```python
from build123d import *

# Parameters (mm, degrees)
CROQUIS1_R              = 9.5
SALIENTE_EXTRUIR1_DEPTH = 6
CROQUIS2_R              = 1.5
CORTAR_EXTRUIR1_DEPTH   = 6
CROQUIS3_R              = 3
CORTAR_EXTRUIR2_DEPTH   = 6
REDONDEO1_R             = 1


with BuildPart() as part:
    # Croquis1 → Saliente-Extruir1 (new body)
    with BuildSketch(Plane(origin=(0, 0, 0), x_dir=(1, 0, 0), z_dir=(0, 1, 0))):
        with BuildLine():
            ThreePointArc((12.5, 0), (0, 12.5), (-12.5, 0))
            Line((-12.5, 0), (-12.5, -16))
            ThreePointArc((-12.5, -16), (-13.085786438, -17.414213562), (-14.5, -18))
            Line((-14.5, -18), (-20.5, -18))
            Line((-20.5, -18), (-20.5, -21))
            Line((-20.5, -21), (-5.5, -21))
            Line((-5.5, -21), (-5.5, -36))
            Line((-5.5, -36), (5.5, -36))
            Line((5.5, -36), (5.5, -21))
            Line((5.5, -21), (20.5, -21))
            Line((20.5, -21), (20.5, -18))
            Line((20.5, -18), (14.5, -18))
            ThreePointArc((14.5, -18), (13.085786438, -17.414213562), (12.5, -16))
            Line((12.5, -16), (12.5, 0))
        make_face()
        with Locations(Location((0, 0, 0), (0, 0, 270))):
            Circle(CROQUIS1_R, mode=Mode.SUBTRACT)
    extrude(amount=SALIENTE_EXTRUIR1_DEPTH)

    # Croquis2 → Cortar-Extruir1 (cut)
    with BuildSketch(Plane.XY.offset(21)):
        with Locations((-16.5, 3)):
            Circle(CROQUIS2_R)
        with Locations((16.5, 3)):
            Circle(CROQUIS2_R)
    extrude(amount=-CORTAR_EXTRUIR1_DEPTH, mode=Mode.SUBTRACT)

    # Croquis3 → Cortar-Extruir2 (cut)
    with BuildSketch(Plane(origin=(0, 0, 18), x_dir=(-1, 0, 0), z_dir=(0, 0, -1))):
        with Locations((-16.5, 3)):
            Circle(CROQUIS3_R)
        with Locations((16.5, 3)):
            Circle(CROQUIS3_R)
    extrude(amount=CORTAR_EXTRUIR2_DEPTH, mode=Mode.SUBTRACT)

    # Redondeo1
    redondeo1_edges = [part.edges().sort_by_distance(p)[0] for p in [
        (5.5, 3, 36),
        (-5.5, 3, 36),
        (0, 6, 36),
        (0, 0, 36),
    ]]
    fillet(redondeo1_edges, radius=REDONDEO1_R)


solid = part.part
```
Model file for the job. Use its own axes, mm. A direction names the side the tool comes from. Coordinates: 2 decimals unless noted, no trailing zeros. Order: outer loops, then holes, each group sorted by start corner. A loop starts at its lowest first (then second) coordinate and runs counter-clockwise, first axis right, second up. Notation, with made-up numbers: (42, 43) -> (92, 43) arc R15 ccw to (92, 65) -> close; hole circle Ø10 at (-15, 84). An arc over 180 degrees is marked (long way). Return JSON: item names as keys, results as strings.
Item 1: Slice it at B-B (x = 0). Write the cut outline in (y, z), then the cut area to 3 significant figures.
Model answer:
{"outline": "(0, -12.5) -> (6, -12.5) -> (6, -9.5) -> (0, -9.5) -> close; (0, 9.5) -> (6, 9.5) -> (6, 35) arc R1 ccw to (5, 36) -> (1, 36) arc R1 ccw to (0, 35) -> close", "area": "177 mm²"}
Item 2: Pin check, flat tips, straight feed: P1, Ø1.8, axis at y = 4, z = 28, coming from the -X side; P2, Ø1, axis at y = 5, z = -5, coming from the -X side; P3, Ø1.5, axis at x = 9.5, y = 0.5, coming from the +Z side. Stop position of each tip, or through.
Model answer:
{"P1": "stops at x = -5.5", "P2": "stops at x = -11.66", "P3": "stops at z = 21"}
Item 3: Wall check: line 1 along X through (y, z) = (2.7, 0); line 2 along X through (y, z) = (4.5, 10.5); line 3 along X through (y, z) = (4.5, -1). Give the ranges that are in metal, low to high. Write a range as from..to.
Model answer:
{"line 1": "x = -12.5..-9.5, 9.5..12.5", "line 2": "x = -12.5..12.5", "line 3": "x = -12.46..-9.45, 9.45..12.46"}
Item 4: Slice it at C-C (x = -16.5). Write the cut outline in (y, z).
Model answer:
{"outline": "(0, 18) -> (1.5, 18) -> (1.5, 21) -> (0, 21) -> close; (4.5, 18) -> (6, 18) -> (6, 21) -> (4.5, 21) -> close"}
Item 5: 3-axis set-ups, long thin cutter, end or side, ignore diameter. For faces 4 (the face through (-13, 3, 21)), 5 (the face through (0, 3, 36)), 6 (the face through (13, 3, 21)): which of +Z, -Z, +X, -X, +Y, -Y reach the whole face in a straight line?
Model answer:
{"face 4": "+Z, -X, +Y, -Y", "face 5": "+Z, +X, -X, +Y, -Y", "face 6": "+Z, +X, +Y, -Y"}
Item 6: Slice it at A-A (y = 3). Write the cut outline in (x, z).
Model answer:
{"outline": "(-20.5, 18) -> (-18, 18) -> (-18, 21) -> (-20.5, 21) -> close; (-15, 18) -> (-13.5, 18) -> (-13.5, 17.73) arc R2 cw to (-12.5, 16) -> (-12.5, 0) arc R12.5 ccw to (12.5, 0) -> (12.5, 16) arc R2 cw to (13.5, 17.73) -> (13.5, 18) -> (15, 18) -> (15, 21) -> (5.5, 21) -> (5.5, 35) arc R1 ccw to (4.5, 36) -> (-4.5, 36) arc R1 ccw to (-5.5, 35) -> (-5.5, 21) -> (-15, 21) -> close; (18, 18) -> (20.5, 18) -> (20.5, 21) -> (18, 21) -> close; hole circle Ø19 at (0, 0)"}
Item 7: Mould opens along Z. For faces 1 (the face through (5.215, 3.042, 35.699)), 2 (the face through (-5.78, 2.96, -7.54)), 3 (the face through (-18, 3, 20)) say: pulls with the +Z half, pulls with the -Z half, needs draft (parallel to the pull), parting line crosses it, or undercut.
Model answer:
{"face 1": "pulls with the +Z half", "face 2": "undercut", "face 3": "needs draft"}
Item 8: Slice it at D-D (z = 13). Write the cut outline in (x, y), then the cut area to 3 significant figures.
Model answer:
{"outline": "(-12.5, 0) -> (12.5, 0) -> (12.5, 6) -> (-12.5, 6) -> close", "area": "150 mm²"}
